The figure shows three views and two pictorial views of one solid part (mm, origin at its lowest corner). Answer the questions. Coordinates: 2 decimals unless noted, no trailing zeros. Loops run counter-clockwise (first coordinate to the right, second up) from the corner with the lowest first, then second, coordinate; pieces in that order, holes last. Notation, with made-up numbers: M 47.25,-5 L 77.25,-5 A21 cw 77.25,31 Z; hole C -1,53.25 d3. An arc over 180 degrees is marked long. One line per item, written item: value. Start each with the question number.
1. Determine the mould class of the marked faces 1, 2 and 3 for opening direction Y: +Y half, -Y half, draft (parallel to the pull), parting line (faces both ways), or undercut.
2. Consider probe 1 along Y at (x, z) = (12.1, 4.5); probe 2 along Y at (x, z) = (1.75, 2.25); probe 3 along Y at (x, z) = (8.75, 1.25). Determine where each line is inside the solid, lowest interval first.
3. Flat-ended cylindrical pins translate along their axes: pin 1 (5 mm diameter, centred on y = 7.5, z = 2, fed in from +X); pin 2 (1.5 mm diameter, centred on y = 3, z = 9.5, fed in from -X); pin 3 (1.5 mm diameter, centred on x = 9.5, z = 6, fed in from -Y). Find the tip coordinate at first contact, or state that the pin passes through.
4. The part is cut by section A-A (y = 12.1). Write down the section's boundary in (x, z).
5. The part is cut by section C-C (z = 7). Write down the section's boundary in (x, y).
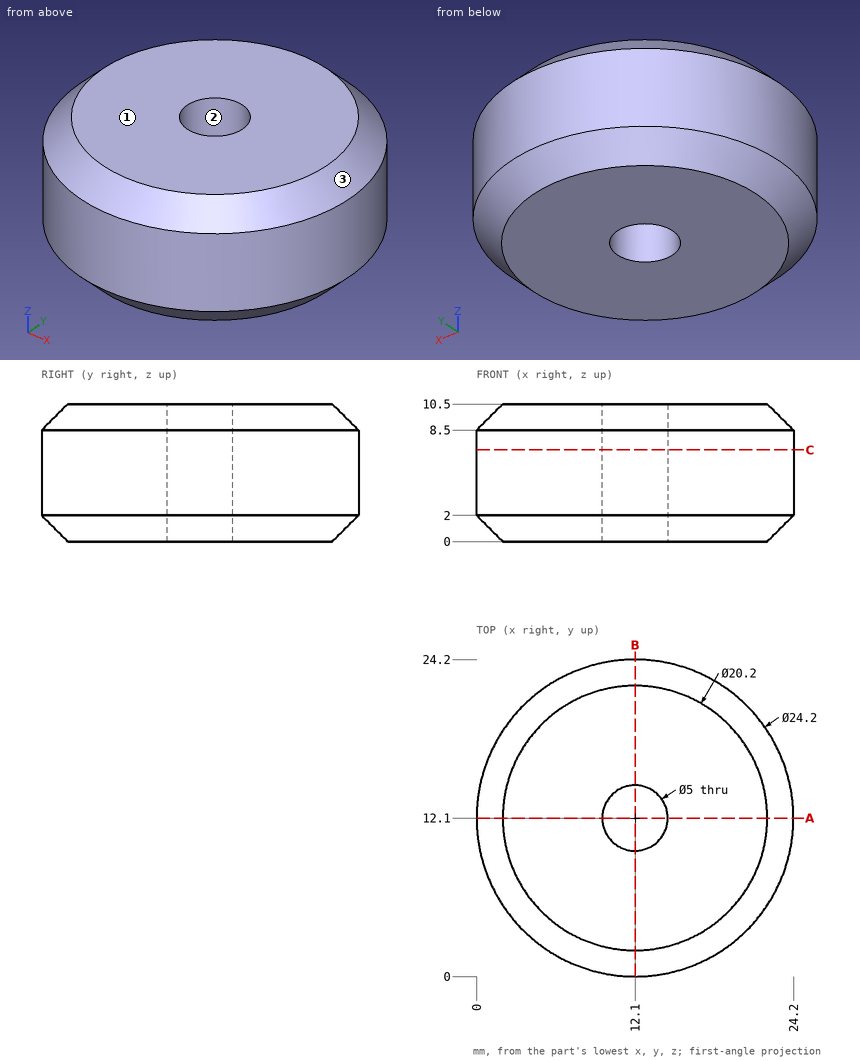
Answer block:
1. face 1: draft
1. face 2: undercut
1. face 3: parting line
2. probe 1: y = 0 to 9.6, 14.6 to 24.2
2. probe 2: y = 5.83 to 18.37
2. probe 3: y = 1.26 to 22.94
3. pin 1: stops at x = 24.02
3. pin 2: stops at x = 4.22
3. pin 3: stops at y = 0.14
4. outline: M 0,2 L 2,0 L 9.6,0 L 9.6,10.5 L 2,10.5 L 0,8.5 Z; M 14.6,0 L 22.2,0 L 24.2,2 L 24.2,8.5 L 22.2,10.5 L 14.6,10.5 Z
5. outline: C 12.1,12.1 d24.2; hole C 12.1,12.1 d5
